Job drawing, mm, ordinate dimensions from the low corner. One solid piece. Coordinates: 2 decimals unless noted, no trailing zeros. Write each loop counter-clockwise with the first axis right and the second up, starting at its lowest first coordinate (ties: lowest second). Pieces come first, ordered by that corner, then holes. Notation, with made-up numbers: (-35.75, -36) - (1.25, -36) arc R24 ccw to (1.25, -16) - close; hole circle Ø5 at (83.25, 23). An arc over 180 degrees is marked (long way). Use a Markdown table: item, result.
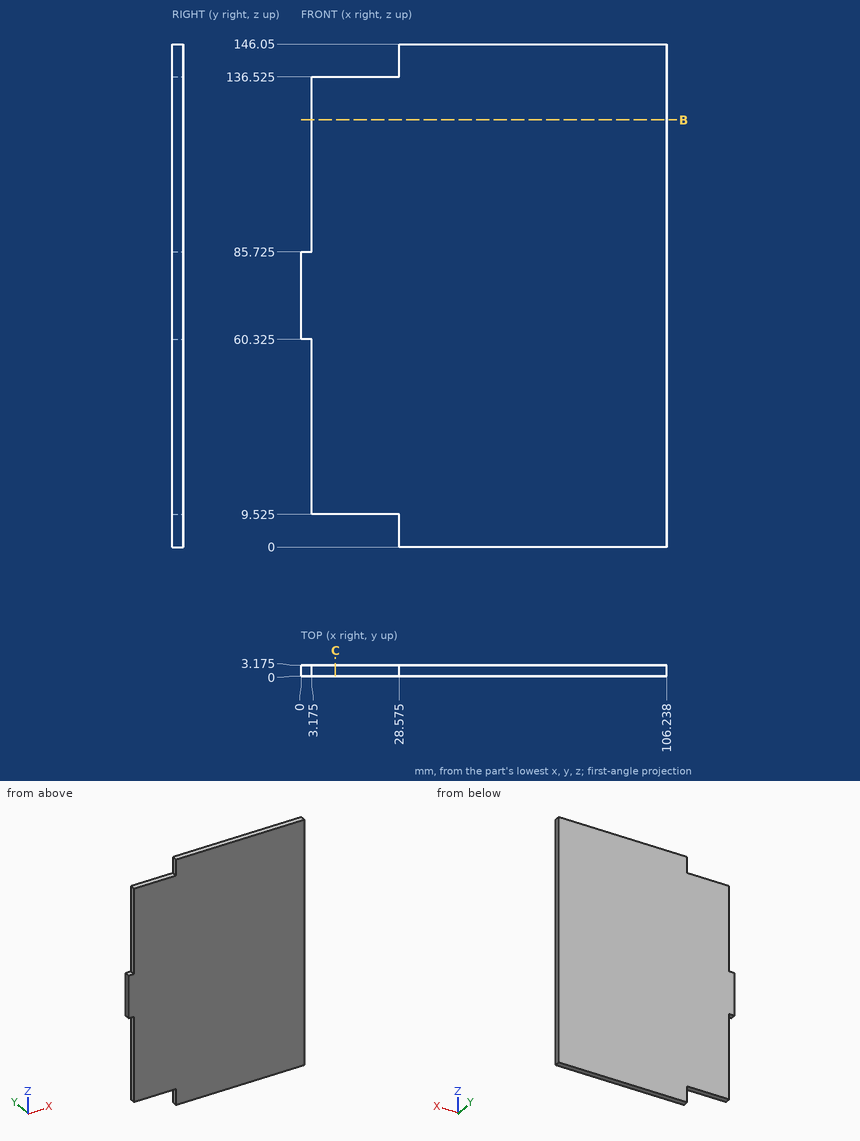
Item 1: Band-saw the part on C-C, the plane x = 10. Give the cut face in (y, z) (1 decimal), then the cut area to 3 significant figures.
From the geometry:
| item | result |
|---|---|
| outline | (0, 9.5) - (3.2, 9.5) - (3.2, 136.5) - (0, 136.5) - close |
| area | 403 mm^2 |
Item 2: Drop flat-ended pins along their axis: P1, Ø3, axis at x = 24.5, z = 97.5, coming from the -Y side; P2, Ø1.6, axis at y = 1.5, z = 103.5, coming from the -X side (1 decimal); P3, Ø1.6, axis at x = 21.5, y = 2, coming from the +Z side (1 decimal); P4, Ø1.6, axis at x = 1, y = 2.5, coming from the +Z side (1 decimal). Give the stop position or say it passes through.
From the geometry:
| item | result |
|---|---|
| P1 | y = 0 |
| P2 | x = 3.2 |
| P3 | z = 136.5 |
| P4 | z = 85.7 |
Item 3: Drill centre lines: probe 1 along X at (y, z) = (2.35, 109) (1 decimal); probe 2 along X at (y, z) = (0.3, 8) (1 decimal); probe 3 along Z at (x, y) = (13.5, 2.65) (1 decimal). Where is each one in solid material? Low to high.
From the geometry:
| item | result |
|---|---|
| probe 1 | 3.2 to 106.2 |
| probe 2 | 28.6 to 106.2 |
| probe 3 | 9.5 to 136.5 |
Item 4: Band-saw the part on B-B, the plane z = 124. Give the cut face in (x, y) (1 decimal), then the cut area to 3 significant figures.
From the geometry:
| item | result |
|---|---|
| outline | (3.2, 0) - (106.2, 0) - (106.2, 3.2) - (3.2, 3.2) - close |
| area | 327 mm^2 |
